For this review, use the dimensioned drawing (mm, ordinates from the lowest corner) and the shaded views. Give positions to 0.01 mm unless a question says otherwise; leave off trailing zeros. Order: outer loops, then holes, each group sorted by start corner. A loop starts at its lowest first (then second) coordinate and runs counter-clockwise, first axis right, second up. Notation, with made-up numbers: M 42,18.25 L 98,18.25 A15 ccw 98,30.25 Z; hole C 57.5,64 d8. An arc over 180 degrees is marked long. One line per question, with ' | ' between items. Start each with the question number.
1. Wall thickness on L1, parallel to Y at x = 38, z = 4.2; L2, parallel to Y at x = 34.5, z = 5.15; L3, parallel to Z at x = 12.5, y = 33: over which ranges is each line inside the solid? List them lowest first.
2. We need section A-A on x = 35. Write out the cut boundary in (y, z), then the cut area to 3 significant figures.
3. The part is to be moulded in two halves that separate along X. For the marked faces 1, 2 and 3, say which applies: +X half, -X half, draft (parallel to the pull), parting line (faces both ways), or undercut.
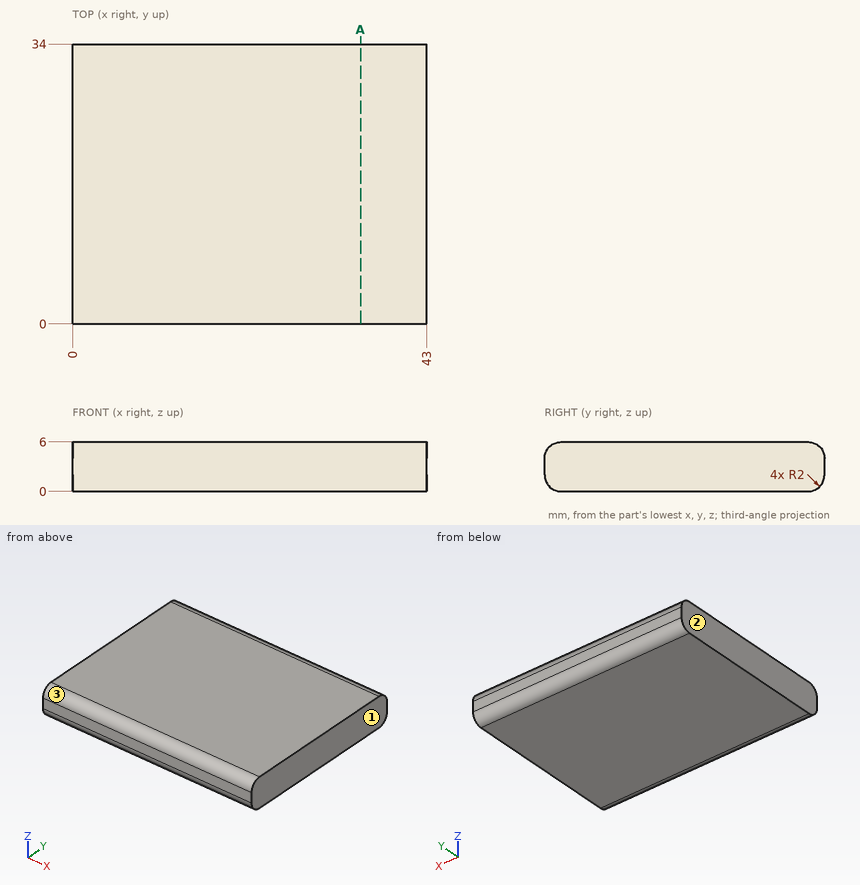
Entries:
1) L1: y = 0.01 to 33.99 | L2: y = 0.36 to 33.64 | L3: z = 0.27 to 5.73
2) outline: M 0,2 A2 ccw 2,0 L 32,0 A2 ccw 34,2 L 34,4 A2 ccw 32,6 L 2,6 A2 ccw 0,4 Z | area: 201 mm^2
3) face 1: +X half | face 2: -X half | face 3: draft
